from build123d import *

# Parameters (mm, degrees)
CUT_EXTRUDE1_DEPTH       = 11
SKETCH4_R                = 2.5
BOSS_EXTRUDE1_DEPTH      = 5
BOSS_EXTRUDE1_DEPTH_BACK = 5
SKETCH5_R                = 1.25
CUT_EXTRUDE2_DEPTH       = 5


with BuildPart() as part:
    # Sketch2 → Revolve2 (revolve)
    with BuildSketch(Plane(origin=(0, 0, 0), x_dir=(0, 0, -1), z_dir=(1, 0, 0))):
        Polygon((-0.947368421, 0), (3.052631579, 20), (-6.947368421, 20), (-2.947368421, 0), align=None)
    revolve(axis=Axis((0, 0, 1.947368421), (0, 0, -1)))

    # Sketch3 → Cut-Extrude1 (cut, through all)
    with BuildSketch(Plane.XY.offset(6.947368421)):
        with BuildLine():
            Line((1.427639009, 3.341779315), (5.437421768, 14.812857935))
            ThreePointArc((5.437421768, 14.812857935), (2.195765142, 15.648221894), (-1.139973889, 15.929319272))
            ThreePointArc((-1.139973889, 15.929319272), (-4.401690999, 15.176078194), (-7.49135707, 13.887616244))
            Line((-7.49135707, 13.887616244), (-1.888958706, 3.104428633))
            ThreePointArc((-1.888958706, 3.104428633), (-0.255193929, 3.565928667), (1.427639009, 3.341779315))
        make_face()
        with BuildLine():
            Line((3.619385709, -0.325098782), (15.768120796, -0.593870567))
            ThreePointArc((15.768120796, -0.593870567), (15.560872146, 2.74726975), (14.797411589, 6.00660996))
            ThreePointArc((14.797411589, 6.00660996), (13.073110736, 8.875922977), (10.892951279, 11.416213388))
            Line((10.892951279, 11.416213388), (2.368766739, 2.755827692))
            ThreePointArc((2.368766739, 2.755827692), (3.312540434, 1.344636408), (3.619385709, -0.325098782))
        make_face()
        with BuildLine():
            Line((0.809264378, -3.542701412), (4.307812822, -15.17989013))
            ThreePointArc((4.307812822, -15.17989013), (7.421382738, -13.950315812), (10.285277197, -12.217030159))
            ThreePointArc((10.285277197, -12.217030159), (12.481317772, -9.690456113), (14.223571198, -6.832008347))
            Line((14.223571198, -6.832008347), (3.352937062, -1.401233452))
            ThreePointArc((3.352937062, -1.401233452), (2.302456507, -2.734897664), (0.809264378, -3.542701412))
        make_face()
        with BuildLine():
            Line((-3.119232818, -1.864411103), (-13.105746054, -8.787817479))
            ThreePointArc((-13.105746054, -8.787817479), (-10.97420537, -11.369039076), (-8.440760697, -13.55714984))
            ThreePointArc((-8.440760697, -13.55714984), (-5.359232128, -14.864954222), (-2.102300837, -15.638626758))
            Line((-2.102300837, -15.638626758), (-0.296537672, -3.621837592))
            ThreePointArc((-0.296537672, -3.621837592), (-1.889544056, -3.03489612), (-3.119232818, -1.864411103))
        make_face()
        with BuildLine():
            Line((-2.737056278, 2.390431982), (-12.407609332, 9.748720242))
            ThreePointArc((-12.407609332, 9.748720242), (-14.203814656, 6.923863244), (-15.501954199, 3.838250768))
            ThreePointArc((-15.501954199, 3.838250768), (-15.793505381, 0.503409163), (-15.52286457, -2.833194526))
            Line((-15.52286457, -2.833194526), (-3.536207423, -0.837185281))
            ThreePointArc((-3.536207423, -0.837185281), (-3.470258956, 0.85922871), (-2.737056278, 2.390431982))
        make_face()
    extrude(amount=-CUT_EXTRUDE1_DEPTH, mode=Mode.SUBTRACT)

    # Sketch4 → Boss-Extrude1 (add, two sides)
    with BuildSketch(Plane.XY.offset(6.947368421)) as boss_extrude1_sk:
        Circle(SKETCH4_R)
    extrude(amount=BOSS_EXTRUDE1_DEPTH)
    extrude(boss_extrude1_sk.sketch, amount=-BOSS_EXTRUDE1_DEPTH_BACK)

    # Sketch5 → Cut-Extrude2 (cut)
    with BuildSketch(Plane.XY.offset(11.947368421)):
        Circle(SKETCH5_R)
    extrude(amount=-CUT_EXTRUDE2_DEPTH, mode=Mode.SUBTRACT)


solid = part.part
Could you check a few things on this model? Use its own coordinates, in mm. A direction names the side the tool comes from. Give positions to 0.01 mm unless a question says otherwise; leave off trailing zeros. Order: outer loops, then holes, each group sorted by start corner. A loop starts at its lowest first (then second) coordinate and runs counter-clockwise, first axis right, second up.
1. Suppose I cut it at C-C (y = -6). Give the number of separate pieces and of enclosed holes in the cut face, plus the area to 3 significant figures.
2. Will these pins go through, and if not, where does the flat tip stop? P1, Ø1.5, axis at y = 15.5, z = 2.5, coming from the +X side; P2, Ø1, axis at y = -11.5, z = -1, coming from the -X side; P3, Ø5, axis at y = -14.5, z = 10, coming from the -X side; P4, Ø8, axis at x = 16, z = 2, coming from the -Y side.
3. For faces 3 (the cylindrical face through (1.34, 2.11, 7.76)), 4 (the cylindrical face through (-15.793, 0.55, 2.006)), which set-ups out of +Z, -Z, +X, -X, +Y, -Y let a thin tool reach every point of the face, with its end or its side?
4. Suppose I cut it at B-B (z = -1.25). List the corners of the cut face in (x, y) for me.
5. Suppose I cut it at A-A (z = 4.5). List the corners of the cut face in (x, y) for me.
6. We'd pull the mould along X, two halves only. Please class faces 1 (the cylindrical face through (3.3, 1.37, 1.97)), 2 (the cylindrical face through (-19.524, -4.336, 2.017)): pulls with the +X half, pulls with the -X half, needs draft (parallel to the pull), parting line crosses it, or undercut.
7. Suppose I cut it at D-D (z = 8.5). List the corners of the cut face in (x, y) for me, plus the area to 3 significant figures.
8. I need wall thicknesses on L1, parallel to Y at x = 0, z = 8.9; L2, parallel to X at y = 11, z = 4; L3, parallel to X at y = 6.5, z = 1.25. Which ranges of each line are inside material? Lowest first, please.
Solved:
1. separate pieces: 3
1. enclosed holes: 0
1. area: 148 mm2
2. P1: stops at x = 13.51
2. P2: stops at x = -16.7
2. P3: passes through
2. P4: stops at y = -16
3. face 3: +Z
3. face 4: +Z, -Z
4. outline: circle Ø40 at (0, 0); hole (-15.52, -2.83) - (-10.79, -2.05) arc R10.99 ccw to (-9.17, -6.06) - (-13.11, -8.79) arc R19.93 ccw to (-8.44, -13.56) arc R19.93 ccw to (-2.1, -15.64) - (-1.39, -10.9) arc R10.99 ccw to (2.93, -10.59) - (4.31, -15.18) arc R19.93 ccw to (10.29, -12.22) arc R19.93 ccw to (14.22, -6.83) - (9.94, -4.69) arc R10.99 ccw to (10.98, -0.49) - (15.77, -0.59) arc R19.93 ccw to (14.8, 6.01) arc R19.93 ccw to (10.89, 11.42) - (7.53, 8) arc R10.99 ccw to (3.86, 10.29) - (5.44, 14.81) arc R19.93 ccw to (-1.14, 15.93) arc R19.93 ccw to (-7.49, 13.89) - (-5.28, 9.63) arc R10.99 ccw to (-8.59, 6.85) - (-12.41, 9.75) arc R19.93 ccw to (-15.5, 3.84) arc R19.93 ccw to start
5. outline: circle Ø40 at (0, 0); circle Ø5 at (0, 0); hole (-15.52, -2.83) - (-7.61, -1.52) arc R7.76 ccw to (-6.52, -4.22) - (-13.11, -8.79) arc R19.93 ccw to (-8.44, -13.56) arc R19.93 ccw to (-2.1, -15.64) - (-0.91, -7.71) arc R7.76 ccw to (2, -7.5) - (4.31, -15.18) arc R19.93 ccw to (10.29, -12.22) arc R19.93 ccw to (14.22, -6.83) - (7.05, -3.25) arc R7.76 ccw to (7.75, -0.42) - (15.77, -0.59) arc R19.93 ccw to (14.8, 6.01) arc R19.93 ccw to (10.89, 11.42) - (5.27, 5.7) arc R7.76 ccw to (2.79, 7.24) - (5.44, 14.81) arc R19.93 ccw to (-1.14, 15.93) arc R19.93 ccw to (-7.49, 13.89) - (-3.79, 6.77) arc R7.76 ccw to (-6.03, 4.89) - (-12.41, 9.75) arc R19.93 ccw to (-15.5, 3.84) arc R19.93 ccw to start
6. face 1: undercut
6. face 2: parting line crosses it
7. outline: circle Ø5 at (0, 0); hole circle Ø2.5 at (0, 0)
7. area: 14.7 mm2
8. L1: y = -2.5 to -1.25, 1.25 to 2.5
8. L2: x = -16.7 to -5.99, 4.1 to 10.48, 11.3 to 16.7
8. L3: x = -18.91 to -14.42, -8.14 to -3.65, 2.53 to 6.05, 14.55 to 18.91
